Read the model definition and answer for the solid it produces. Units are mm, in the model's axes. A direction names the side the tool comes from. Round coordinates to 2 decimals unless told otherwise and drop trailing zeros. Order: outer loops, then holes, each group sorted by start corner. A loop starts at its lowest first (then second) coordinate and runs counter-clockwise, first axis right, second up. Notation, with made-up numbers: (21, 40.5) -> (28, 40.5) arc R12 cw to (28, 46.5) -> close; hole circle Ø11 at (-29, 7.5). An arc over 180 degrees is marked (long way). Use a Markdown table: item, result. Add a question column.
1. For faces 1 (the face through (-7.939, -10.477, 6.084)), 2 (the face through (-4.75, 1, 6)), determine the directions among +Z, -Z, +X, -X, +Y, -Y from which every point of the face is accessible in a straight line to the end or side of a thin tool.
2. Consider L1, parallel to Y at x = 7.5, z = 7.5 (3 decimals); L2, parallel to X at y = -7, z = 6; L3, parallel to X at y = -8, z = 5.75. Determine where each line is inside the solid, lowest interval first. Write a range as [from, to].
3. Section C-C, the plane z = 1.75 is taken. Give the vertices of the cut face in (x, y) (3 decimals), then the cut area to 3 significant figures.
4. The mould has two halves that part along Y. Classify faces 3 (the face through (7.061, -10.477, 6.084)), 4 (the face through (0, -7, 0)), 5 (the face through (14.4, -16.43, 6.08)): +Y half, -Y half, draft (parallel to the pull), parting line (faces both ways), or undercut.
5. Section B-B, the plane y = -8.5 is taken. Give the vertices of the cut face in (x, z) (3 decimals).
6. Section A-A, the plane x = -7.5 is taken. Give the vertices of the cut face in (y, z) (3 decimals), then the cut area to 3 significant figures.
```python
from build123d import *

# Parameters (mm, degrees)
EXTRUDE_1_DEPTH          = 12
FILLET_1_R               = 2
SKETCH_2_R               = 2.025
CUT_EXTRUDE_1_DEPTH      = 1
CUT_EXTRUDE_1_DEPTH_BACK = 13


with BuildPart() as part:
    # 草图1 → 凸台-拉伸1 (new body)
    with BuildSketch(Plane.XY):
        Polygon((4.75, 0), (-4.75, 0), (-4.75, 3), (-15, 3), (-15, -17), (15, -17), (15, 3), (4.75, 3), align=None)
    extrude(amount=EXTRUDE_1_DEPTH)

    # 圆角1
    fillet_1_edges = [part.edges().sort_by_distance(p)[0] for p in [
        (15, 3, 6),
        (15, -17, 6),
        (-15, -17, 6),
        (-15, 3, 6),
    ]]
    fillet(fillet_1_edges, radius=FILLET_1_R)

    # 草图2 → 切除-拉伸1 (cut, two sides)
    with BuildSketch(Plane.XY.offset(12)) as cut_extrude_1_sk:
        with Locations((-7.5, -8.5)):
            Circle(SKETCH_2_R)
        with Locations((7.5, -8.5)):
            Circle(SKETCH_2_R)
    extrude(amount=CUT_EXTRUDE_1_DEPTH, mode=Mode.SUBTRACT)
    extrude(cut_extrude_1_sk.sketch, amount=-CUT_EXTRUDE_1_DEPTH_BACK, mode=Mode.SUBTRACT)


solid = part.part
```
Verdict:
| question | item | result |
|---|---|---|
| 1 | face 1 | +Z, -Z |
| 1 | face 2 | +Z, -Z, +Y |
| 2 | L1 | y = [-17, -10.525], [-6.475, 3] |
| 2 | L2 | x = [-15, -8.86], [-6.14, 6.14], [8.86, 15] |
| 2 | L3 | x = [-15, -9.46], [-5.54, 5.54], [9.46, 15] |
| 3 | outline | (-15, -15) arc R2 ccw to (-13, -17) -> (13, -17) arc R2 ccw to (15, -15) -> (15, 1) arc R2 ccw to (13, 3) -> (4.75, 3) -> (4.75, 0) -> (-4.75, 0) -> (-4.75, 3) -> (-13, 3) arc R2 ccw to (-15, 1) -> close; hole circle Ø4.05 at (-7.5, -8.5); hole circle Ø4.05 at (7.5, -8.5) |
| 3 | area | 542 mm2 |
| 4 | face 3 | undercut |
| 4 | face 4 | draft |
| 4 | face 5 | -Y half |
| 5 | outline | (-15, 0) -> (-9.525, 0) -> (-9.525, 12) -> (-15, 12) -> close; (-5.475, 0) -> (5.475, 0) -> (5.475, 12) -> (-5.475, 12) -> close; (9.525, 0) -> (15, 0) -> (15, 12) -> (9.525, 12) -> close |
| 6 | outline | (-17, 0) -> (-10.525, 0) -> (-10.525, 12) -> (-17, 12) -> close; (-6.475, 0) -> (3, 0) -> (3, 12) -> (-6.475, 12) -> close |
| 6 | area | 191 mm2 |
